Geometry: final body of the model. Coordinates: model frame, mm. Give positions to 0.01 mm unless a question says otherwise; leave off trailing zeros. Order: outer loops, then holes, each group sorted by start corner. A loop starts at its lowest first (then second) coordinate and runs counter-clockwise, first axis right, second up. Notation, with made-up numbers: (53, 68) - (79, 68) arc R28 cw to (79, 98) - close; hole circle Ø8 at (-8.75, 4). An arc over 180 degrees is marked (long way). Use one line per item in the form item = value.
from build123d import *

# Parameters (mm, degrees)
F0_W     = 355.6
F0_H     = 304.8
F1_DEPTH = 25.4
F2_W     = 355.6
F2_H     = 304.8
F3_DEPTH = 88.9
F4_R     = 25.4


with BuildPart() as f1:
    # F0 (on Top) → F1 (new body)
    with BuildSketch(Plane.XY):
        Rectangle(F0_W, F0_H)
    extrude(amount=F1_DEPTH)

    # F2 (on face) → F3 (join)
    with BuildSketch(Plane.XY.offset(25.4)):
        Rectangle(F2_W, F2_H)
    extrude(amount=F3_DEPTH)

    # F4
    f4_edges = [f1.edges().sort_by_distance(p)[0] for p in [
        (-177.8, 0, 114.3),
        (0, -152.4, 114.3),
        (177.8, 0, 114.3),
        (0, 152.4, 114.3),
    ]]
    fillet(f4_edges, radius=F4_R)


solid = f1.part
(1) Ray query, line 1 along Z through (x, y) = (-93, -128); line 2 along Y through (x, z) = (-45, 89); line 3 along Y through (x, z) = (106.5, 101.5). Return the intervals inside material, ascending.
Computed values:
line_1 = 0 to 114.28
line_2 = -152.4 to 152.4
line_3 = -149.05 to 149.05
(2) Contact query for flat-ended pins moving along their axis: pin 1 Ø1 at (y, z) = (0.5, 101.5) entering from +X; pin 2 Ø1 at (y, z) = (-93, 91) entering from -X; pin 3 Ø4 at (x, z) = (118, 97.5) entering from +Y. Output: stop coordinate, or through.
Computed values:
pin_1 = 174.73
pin_2 = -177.75
pin_3 = 151.53
(3) Cut plane A-A on z = 104. Output: boundary loops of the cut face in (x, y).
Computed values:
outline = (-172.82, -147.42) - (172.82, -147.42) - (172.82, 147.42) - (-172.82, 147.42) - close
